Geometry: final body of the model. Coordinates: model frame, mm. Face numbers are marked on the shaded views. A direction names the side the tool comes from. Coordinates: 2 decimals unless noted, no trailing zeros. Loops run counter-clockwise (first coordinate to the right, second up) from the corner with the lowest first, then second, coordinate; pieces in that order, holes last. Notation, with made-up numbers: (59.25, 81) - (105.25, 81) arc R29 cw to (105.25, 101) - close; hole circle Ø8 at (62, -34.5). An arc over 180 degrees is marked (long way). Answer in a Markdown table with one row per item.
from build123d import *

# Parameters (mm, degrees)
BOSS_EXTRUDE1_DEPTH = 25.4
CUT_EXTRUDE1_DEPTH  = 5.08
SKETCH3_OUTSIDE_W   = 13.788
SKETCH3_OUTSIDE_H   = 14.77
SKETCH3_OUTSIDE_R   = 3.175
CUT_EXTRUDE2_DEPTH  = 13.7


with BuildPart() as part:
    # Sketch1 → Boss-Extrude1 (new body)
    with BuildSketch(Plane.XY):
        Polygon((0, 3.666174209), (-3.175, 1.833087105), (-3.175, -1.833087105), (0, -3.666174209), (3.175, -1.833087105), (3.175, 1.833087105), align=None)
    extrude(amount=-BOSS_EXTRUDE1_DEPTH)

    # Sketch2 → Cut-Extrude1 (cut)
    with BuildSketch(Plane.XY):
        with BuildLine():
            Line((-1.117311326, -0.62484), (1.117311326, -0.62484))
            ThreePointArc((1.117311326, -0.62484), (0, 1.28016), (-1.117311326, -0.62484))
        make_face()
    extrude(amount=-CUT_EXTRUDE1_DEPTH, mode=Mode.SUBTRACT)

    # Sketch3 outside → Cut-Extrude2 (cut, through all)
    with BuildSketch(Plane.XY.offset(-12.7)):
        Rectangle(SKETCH3_OUTSIDE_W, SKETCH3_OUTSIDE_H)
        Circle(SKETCH3_OUTSIDE_R, mode=Mode.SUBTRACT)
    extrude(amount=-CUT_EXTRUDE2_DEPTH, mode=Mode.SUBTRACT)


solid = part.part
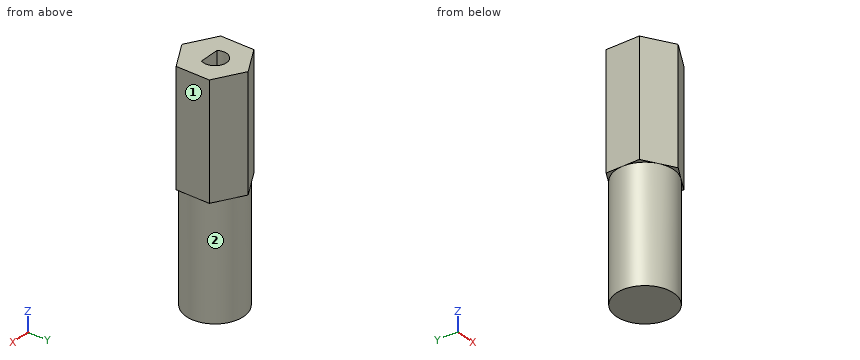
(1) Cut plane A-A on z = -2.75. Output: boundary loops of the cut face in (x, y) (3 decimals).
Verdict:
| item | result |
|---|---|
| outline | (-3.175, -1.833) - (0, -3.666) - (3.175, -1.833) - (3.175, 1.833) - (0, 3.666) - (-3.175, 1.833) - close; hole (-1.117, -0.625) - (1.117, -0.625) arc R1.28 ccw (long way) to start |
(2) Ray query, probe 1 along X at (y, z) = (0, -3.75) (3 decimals); probe 2 along Y at (x, z) = (2.75, -22.5). Return the intervals inside material, ascending.
Verdict:
| item | result |
|---|---|
| probe 1 | x = -3.175 to -1.28, 1.28 to 3.175 |
| probe 2 | y = -1.59 to 1.59 |
(3) Cut plane C-C on y = -2.5. Output: boundary loops of the cut face in (x, z), then the cut area to 3 significant figures.
Verdict:
| item | result |
|---|---|
| outline | (-2.02, -12.7) - (-1.96, -12.7) - (-1.96, -25.4) - (1.96, -25.4) - (1.96, -12.7) - (2.02, -12.7) - (2.02, 0) - (-2.02, 0) - close |
| area | 101 mm² |
(4) Access query for the marked faces 1 and 2. Directions: +Z, -Z, +X, -X, +Y, -Y. A direction counts if a zero-diameter tool reaches every point of the face in a straight line with its end or side. Return the directions, or none.
Verdict:
| item | result |
|---|---|
| face 1 | +Z, -Z, +X, +Y, -Y |
| face 2 | -Z |
(5) Cut plane B-B on x = -2. Output: boundary loops of the cut face in (y, z), then the cut area to 3 significant figures.
Verdict:
| item | result |
|---|---|
| outline | (-2.51, -12.7) - (-2.47, -12.7) - (-2.47, -25.4) - (2.47, -25.4) - (2.47, -12.7) - (2.51, -12.7) - (2.51, 0) - (-2.51, 0) - close |
| area | 126 mm² |
(6) Cut plane D-D on z = -5.75. Output: boundary loops of the cut face in (x, y) (3 decimals), then the cut area to 3 significant figures.
Verdict:
| item | result |
|---|---|
| outline | (-3.175, -1.833) - (0, -3.666) - (3.175, -1.833) - (3.175, 1.833) - (0, 3.666) - (-3.175, 1.833) - close |
| area | 34.9 mm² |
(7) First-contact query: pin 1 Ø1 at (x, z) = (2, -17.5) entering from +Y; pin 2 Ø2 at (x, z) = (0.5, -8) entering from +Y. Flat tips, straight axial feed; report the tip coordinate or a pass-through.
Verdict:
| item | result |
|---|---|
| pin 1 | stops at y = 2.8 |
| pin 2 | stops at y = 3.67 |
